Geometry check sheet. Reference: the model listing, model coordinates, mm. Coordinates: 2 decimals unless noted, no trailing zeros. Write each loop counter-clockwise with the first axis right and the second up, starting at its lowest first coordinate (ties: lowest second). Pieces come first, ordered by that corner, then holes. Notation, with made-up numbers: (50.25, 22.25) - (93.25, 22.25) arc R13 ccw to (93.25, 35.25) - close; hole circle Ø4 at (40, 73). An arc over 180 degrees is marked (long way). Answer as a JSON object with one key per item and string values. Group by question number.
from build123d import *

# Parameters (mm, degrees)
SALIENTE_EXTRUIR1_DEPTH = 3


with BuildPart() as part:
    # Croquis1 → Saliente-Extruir1 (new body)
    with BuildSketch(Plane(origin=(0, 0, 0), x_dir=(1, 0, 0), z_dir=(0, 1, 0))):
        Polygon((0, 200), (0, 203.1), (-3.1, 203.1), (-3.1, 180), (0, 180), (0, 159.996339437), (-2.9, 159.996339437), (-2.9, 139.996339437), (0, 139.996339437), (0, 119.996339437), (-2.9, 119.996339437), (-2.9, 99.996339437), (0, 99.996339437), (0, 80), (-2.9, 80), (-2.9, 60), (0, 60), (0, 40), (-3.1, 40), (-3.1, 20), (0, 20), (0, 0), (-3.1, 0), (-3.1, -3.1), (20, -3.1), (20, 0), (40, 0), (40, -3.1), (60, -3.1), (60, 0), (80, 0), (80, -3.1), (100, -3.1), (100, 0), (120, 0), (120, -3.1), (140, -3.1), (140, 0), (160, 0), (160, -3.1), (180, -3.1), (180, 0), (200, 0), (200, -3.1), (220, -3.1), (220, 0), (240, 0), (240, -3.1), (260, -3.1), (260, 0), (280, 0), (280, -3.1), (300, -3.1), (300, 0), (320, 0), (320, -3.1), (340, -3.1), (340, 0), (360, 0), (360, -3.1), (380, -3.1), (380, 0), (400, 0), (400, -3.1), (420, -3.1), (420, 0), (440, 0), (440, -3.1), (460, -3.1), (460, 0), (480, 0), (480, -3.1), (483.1, -3.1), (483.1, 20), (480, 20), (480, 39.996339437), (483.1, 39.996339437), (483.1, 60), (480, 60), (480, 79.996339437), (483.1, 79.996339437), (483.1, 100), (480, 100), (480, 119.996339437), (483.1, 119.996339437), (483.1, 140), (480, 140), (480, 159.996339437), (483.1, 159.996339437), (483.1, 180), (480, 180), (480, 200), (483.1, 200), (483.1, 203.1), (460, 203.1), (460, 200), (440, 200), (440, 203.1), (420, 203.1), (420, 200), (400, 200), (400, 203.1), (380, 203.1), (380, 200), (360, 200), (360, 203.1), (340, 203.1), (340, 200), (320, 200), (320, 203.1), (300, 203.1), (300, 200), (280, 200), (280, 203.1), (260, 203.1), (260, 200), (240, 200), (240, 203.1), (220, 203.1), (220, 200), (200, 200), (200, 203.1), (180, 203.1), (180, 200), (160, 200), (160, 203.1), (140, 203.1), (140, 200), (120, 200), (120, 203.1), (100, 203.1), (100, 200), (80, 200), (80, 203.1), (60, 203.1), (60, 200), (40, 200), (40, 203.1), (20, 203.1), (20, 200), align=None)
    extrude(amount=SALIENTE_EXTRUIR1_DEPTH)


solid = part.part
(1) Material ranges on L1, parallel to X at y = 2.5, z = -19.5; L2, parallel to X at y = 0.9, z = -186; L3, parallel to Z at x = 91.5, y = 0.7, recorded low to high. Write a range as [from, to].
(2) Gauge pin test, flat ends, axial feed: pin 1 (1 mm diameter, centred on y = 0.5, z = -49, fed in from -X); pin 2 (1 mm diameter, centred on y = 1.5, z = -63.5, fed in from +X); pin 3 (1.5 mm diameter, centred on x = 107.5, y = 1, fed in from +Z). Record the tip position at first contact, or that the pin passes through.
(3) Section check A-A (x = 148). Record the cut outline in (y, z).
Conclusion:
{
 "1": {"L1": "x = [0, 483.1]", "L2": "x = [-3.1, 480]", "L3": "z = [-200, 3.1]"},
 "2": {"pin 1": "stops at x = 0", "pin 2": "stops at x = 480", "pin 3": "stops at z = 0"},
 "3": {"outline": "(0, -203.1) - (3, -203.1) - (3, 0) - (0, 0) - close"}
}
